Model file for the job. Use its own axes, mm. A direction names the side the tool comes from. Round coordinates to 2 decimals unless told otherwise and drop trailing zeros. Loops run counter-clockwise (first coordinate to the right, second up) from the corner with the lowest first, then second, coordinate; pieces in that order, holes last. Notation, with made-up numbers: (41, 37) - (60, 37) arc R19 ccw to (60, 41) - close; hole circle Ø5 at (12.25, 37.5). An arc over 180 degrees is marked (long way). Answer as a JSON object with one key per item and string values.
from build123d import *

# Parameters (mm, degrees)
SKETCH1_R           = 3
SKETCH1_R_2         = 4
BOSS_EXTRUDE1_DEPTH = 1


with BuildPart() as part:
    # Sketch1 → Boss-Extrude1 (new body)
    with BuildSketch(Plane(origin=(0, 0, 0), x_dir=(1, 0, 0), z_dir=(0, 1, 0))):
        with BuildLine():
            Line((-37.239092363, -64.5), (-260.820835382, -64.5))
            ThreePointArc((-260.820835382, -64.5), (-437.239092363, 0), (-260.820835382, 64.5))
            Line((-260.820835382, 64.5), (-37.239092363, 64.5))
            Line((-37.239092363, 64.5), (74.551779147, 258.127469277))
            ThreePointArc((74.551779147, 258.127469277), (218.619546181, 378.660161514), (186.269056235, 193.627469277))
            Line((186.269056235, 193.627469277), (74.478184725, 0))
            Line((74.478184725, 0), (186.269056235, -193.627469277))
            ThreePointArc((186.269056235, -193.627469277), (218.619546181, -378.660161514), (74.551779147, -258.127469277))
            Line((74.551779147, -258.127469277), (-37.239092363, -64.5))
        make_face()
        with Locations((-337.239092363, 85)):
            Circle(SKETCH1_R, mode=Mode.SUBTRACT)
        with Locations((-263.626933041, 42.5)):
            Circle(SKETCH1_R, mode=Mode.SUBTRACT)
        with Locations((-263.626933041, -42.5)):
            Circle(SKETCH1_R, mode=Mode.SUBTRACT)
        with Locations((-337.239092363, -85)):
            Circle(SKETCH1_R, mode=Mode.SUBTRACT)
        with Locations((-410.851251684, -42.5)):
            Circle(SKETCH1_R, mode=Mode.SUBTRACT)
        with Locations((-410.851251684, 42.5)):
            Circle(SKETCH1_R, mode=Mode.SUBTRACT)
        with Locations((168.619546181, 207.057621135)):
            Circle(SKETCH1_R, mode=Mode.SUBTRACT)
        with Locations((242.231705503, 249.557621135)):
            Circle(SKETCH1_R, mode=Mode.SUBTRACT)
        with Locations((242.231705503, 334.557621135)):
            Circle(SKETCH1_R, mode=Mode.SUBTRACT)
        with Locations((168.619546181, 377.057621135)):
            Circle(SKETCH1_R, mode=Mode.SUBTRACT)
        with Locations((95.00738686, 334.557621135)):
            Circle(SKETCH1_R, mode=Mode.SUBTRACT)
        with Locations((95.00738686, 249.557621135)):
            Circle(SKETCH1_R, mode=Mode.SUBTRACT)
        with Locations((95.00738686, -249.557621135)):
            Circle(SKETCH1_R, mode=Mode.SUBTRACT)
        with Locations((95.00738686, -334.557621135)):
            Circle(SKETCH1_R, mode=Mode.SUBTRACT)
        with Locations((168.619546181, -377.057621135)):
            Circle(SKETCH1_R, mode=Mode.SUBTRACT)
        with Locations((242.231705503, -334.557621135)):
            Circle(SKETCH1_R, mode=Mode.SUBTRACT)
        with Locations((242.231705503, -249.557621135)):
            Circle(SKETCH1_R, mode=Mode.SUBTRACT)
        with Locations((168.619546181, -207.057621135)):
            Circle(SKETCH1_R, mode=Mode.SUBTRACT)
        with Locations((-45, -25)):
            Circle(SKETCH1_R_2, mode=Mode.SUBTRACT)
        with Locations((-45, 25)):
            Circle(SKETCH1_R_2, mode=Mode.SUBTRACT)
        with Locations((44.150635095, 26.47114317)):
            Circle(SKETCH1_R_2, mode=Mode.SUBTRACT)
        with Locations((0.849364905, 51.47114317)):
            Circle(SKETCH1_R_2, mode=Mode.SUBTRACT)
        with Locations((0.849364905, -51.47114317)):
            Circle(SKETCH1_R_2, mode=Mode.SUBTRACT)
        with Locations((44.150635095, -26.47114317)):
            Circle(SKETCH1_R_2, mode=Mode.SUBTRACT)
        with BuildLine():
            Line((-427.239092363, -5), (-427.239092363, 5))
            ThreePointArc((-427.239092363, 5), (-422.239092363, 10), (-417.239092363, 5))
            Line((-417.239092363, 5), (-417.239092363, -5))
            ThreePointArc((-417.239092363, -5), (-422.239092363, -10), (-427.239092363, -5))
        make_face(mode=Mode.SUBTRACT)
        with BuildLine():
            Line((209.289419162, 372.499907476), (217.9496732, 367.499907476))
            ThreePointArc((217.9496732, 367.499907476), (219.779800219, 360.669780457), (212.9496732, 358.839653438))
            Line((212.9496732, 358.839653438), (204.289419162, 363.839653438))
            ThreePointArc((204.289419162, 363.839653438), (202.459292144, 370.669780457), (209.289419162, 372.499907476))
        make_face(mode=Mode.SUBTRACT)
        with BuildLine():
            Line((217.9496732, -367.499907476), (209.289419162, -372.499907476))
            ThreePointArc((209.289419162, -372.499907476), (202.459292144, -370.669780457), (204.289419162, -363.839653438))
            Line((204.289419162, -363.839653438), (212.9496732, -358.839653438))
            ThreePointArc((212.9496732, -358.839653438), (219.779800219, -360.669780457), (217.9496732, -367.499907476))
        make_face(mode=Mode.SUBTRACT)
    extrude(amount=BOSS_EXTRUDE1_DEPTH)


solid = part.part
1) Slice it at A-A on x = -170. List the corners of the cut face in (y, z), then the cut area to 3 significant figures.
Values follow:
{"outline": "(0, -64.5) - (1, -64.5) - (1, 64.5) - (0, 64.5) - close", "area": "129 mm²"}
2) Slice it at B-B on y = 0.5. Count the separate pieces of the cut face and the enclosed holes in it, then the cut area to 3 significant figures.
Values follow:
{"separate pieces": "1", "enclosed holes": "27", "area": "180,000 mm²"}
3) Probe probe 1 along X at (y, z) = (0.4, 85); probe 2 along X at (y, z) = (0.55, 26.5); probe 3 along Z at (x, y) = (184, 0.75). List the from-to ranges inside material, lowest first.
Values follow:
{"probe 1": "-389.92 to -340.24, -334.24 to -284.56, -25.4 to 123.55", "probe 2": "-433.66 to -48.71, -41.29 to 40.15, 48.15 to 89.78", "probe 3": "-390.87 to -189.7, 189.7 to 390.87"}
4) Two-plate mould, pull along Z, no slides. Class faces 1 (the cylindrical face through (221.55, 0.49, 376.9)), 2 (the flat face through (-4, 0, -2)), 3 (the cylindrical face through (-437.18, 0.49, 3.42)): pulls with the +Z half, pulls with the -Z half, needs draft (parallel to the pull), parting line crosses it, or undercut.
Values follow:
{"face 1": "undercut", "face 2": "needs draft", "face 3": "parting line crosses it"}
5) Drop flat-ended pins along their axis: P1, Ø5.5, axis at x = -337.24, z = 85, coming from the +Y side; P2, Ø0.5, axis at x = -156.5, y = 0.5, coming from the -Z side. Give the stop position or say it passes through.
Values follow:
{"P1": "through", "P2": "z = -64.5"}
6) Slice it at C-C on z = -319.5. List the corners of the cut face in (x, y), then the cut area to 3 significant figures.
Values follow:
{"outline": "(72.46, 0) - (264.78, 0) - (264.78, 1) - (72.46, 1) - close", "area": "192 mm²"}
7) Tool access for faces 4 (the flat face through (131.156, 0.493, -98.169)), 5 (the flat face through (-4, 1, -2)): list every direction of +Z, -Z, +X, -X, +Y, -Y with a clear straight run to the whole face (end or side of a thin tool).
Values follow:
{"face 4": "+X, +Y, -Y", "face 5": "+Z, -Z, +X, -X, +Y"}
